Answer from the drawing. Dimensions are ordinates in mm from the lowest x, y and z of the part. Give positions to 0.01 mm unless a question says otherwise; leave off trailing zeros. Write each loop counter-clockwise with the first axis right and the second up, starting at its lowest first coordinate (ties: lowest second). Pieces come first, ordered by that corner, then holes.
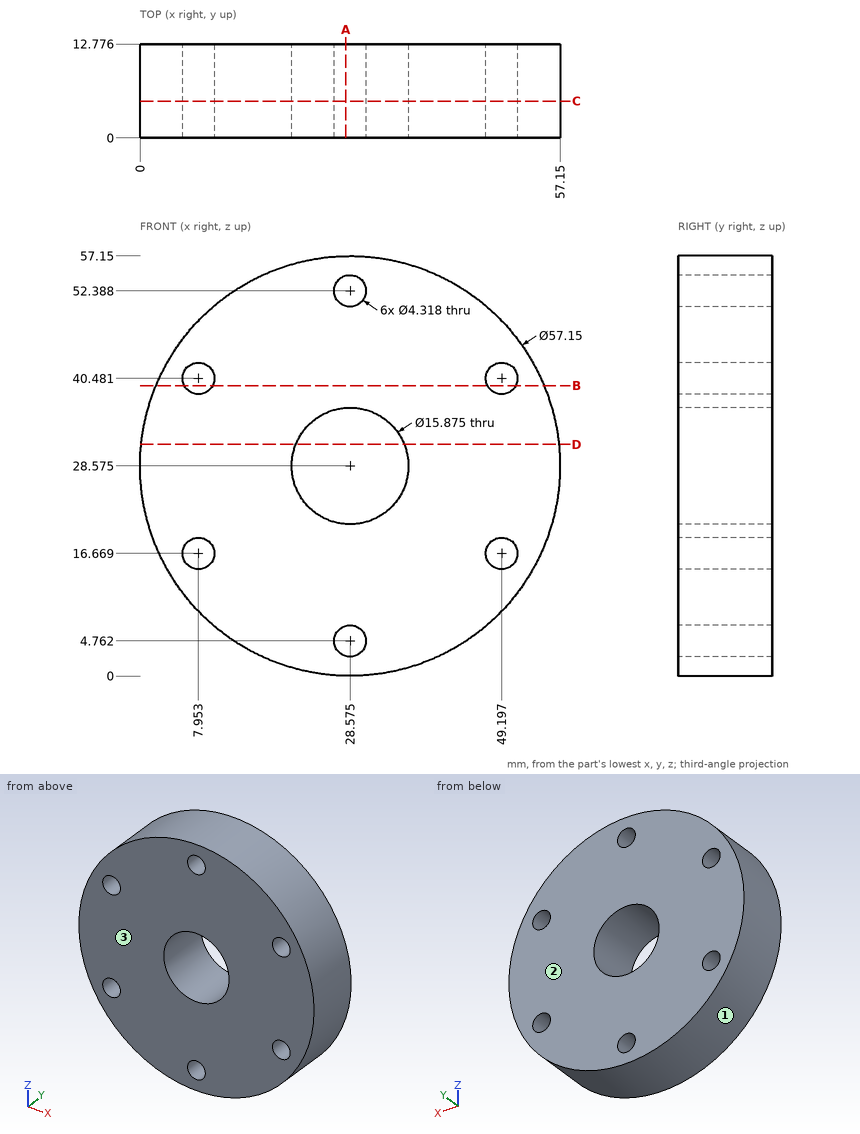
Item 1: A cutting plane is placed at C-C, the plane y = 5. Count the separate pieces of the cut face and the enclosed holes in it, plus the area to 3 significant figures.
Conclusion:
separate pieces: 1
enclosed holes: 7
area: 2,280 mm2
Item 2: A cutting plane is placed at D-D, the plane z = 31.5. Give the vertices of the cut face in (x, y).
Conclusion:
outline: (0.15, 0) - (21.2, 0) - (21.2, 12.78) - (0.15, 12.78) - close; (35.95, 0) - (57, 0) - (57, 12.78) - (35.95, 12.78) - close
Item 3: A cutting plane is placed at A-A, the plane x = 28. Give the vertices of the cut face in (y, z) (1 decimal).
Conclusion:
outline: (0, 0) - (12.8, 0) - (12.8, 2.7) - (0, 2.7) - close; (0, 6.8) - (12.8, 6.8) - (12.8, 20.7) - (0, 20.7) - close; (0, 36.5) - (12.8, 36.5) - (12.8, 50.3) - (0, 50.3) - close; (0, 54.5) - (12.8, 54.5) - (12.8, 57.1) - (0, 57.1) - close
Item 4: Consider probe 1 along Z at (x, y) = (50, 5.5) (1 decimal); probe 2 along Z at (x, y) = (51, 5.5) (1 decimal); probe 3 along X at (y, z) = (0.5, 28.5). Determine where each line is inside the solid, lowest interval first.
Conclusion:
probe 1: z = 9.7 to 14.7, 18.7 to 38.5, 42.5 to 47.5
probe 2: z = 10.9 to 15.5, 17.9 to 39.3, 41.7 to 46.3
probe 3: x = 0 to 20.64, 36.51 to 57.15
Item 5: Determine the mould class of the marked faces 1, 2 and 3 for opening direction Y: pulls with the +Y half, pulls with the -Y half, needs draft (parallel to the pull), parting line crosses it, or undercut.
Conclusion:
face 1: needs draft
face 2: pulls with the +Y half
face 3: pulls with the -Y half
Item 6: Each of these flat-tipped pins is pushed along its axis until it touches: P1, Ø3, axis at y = 3.5, z = 24.5, coming from the +X side; P2, Ø1, axis at y = 10.5, z = 33.5, coming from the +X side (1 decimal); P3, Ø2, axis at x = 51, y = 5.5, coming from the +Z side; P4, Ø12.5, axis at x = 28.575, z = 28.575, coming from the +Y side. Where does it stop, or does it pass through?
Conclusion:
P1: stops at x = 57.03
P2: stops at x = 56.8
P3: stops at z = 47.48
P4: passes through
Item 7: A cutting plane is placed at B-B, the plane z = 39.5. Give the vertices of the cut face in (x, y) (1 decimal).
Conclusion:
outline: (2.2, 0) - (6, 0) - (6, 12.8) - (2.2, 12.8) - close; (9.9, 0) - (47.3, 0) - (47.3, 12.8) - (9.9, 12.8) - close; (51.1, 0) - (55, 0) - (55, 12.8) - (51.1, 12.8) - close
